from build123d import *

# Parameters (mm, degrees)
SKETCH_1_R          = 1.6
EXTRUDE_1_DEPTH     = 3
SKETCH_2_R          = 1.6
CUT_EXTRUDE_1_DEPTH = 4
SKETCH_3_R          = 1.6
CUT_EXTRUDE_2_DEPTH = 4
SKETCH_4_W          = 38
SKETCH_4_H          = 12.5
CUT_EXTRUDE_3_DEPTH = 4
FILLET_1_R          = 3


with BuildPart() as part:
    # 草图1 → 凸台-拉伸1 (new body)
    with BuildSketch(Plane.XY):
        Polygon((-40, 0), (-48, 25.855555556), (-48, 50), (5, 50), (5, 25.855555556), (0, 0), align=None)
        with Locations((-44, 46)):
            Circle(SKETCH_1_R, mode=Mode.SUBTRACT)
        with Locations((1, 46)):
            Circle(SKETCH_1_R, mode=Mode.SUBTRACT)
        with Locations((1, 27.5)):
            Circle(SKETCH_1_R, mode=Mode.SUBTRACT)
        with Locations((-44, 27.5)):
            Circle(SKETCH_1_R, mode=Mode.SUBTRACT)
    extrude(amount=EXTRUDE_1_DEPTH)

    # 草图2 → 切除-拉伸1 (cut, through all)
    with BuildSketch(Plane.XY.offset(3)):
        with Locations((-5, 3)):
            Circle(SKETCH_2_R)
        with Locations((-15, 3)):
            Circle(SKETCH_2_R)
        with Locations((-25, 3)):
            Circle(SKETCH_2_R)
        with Locations((-35, 3)):
            Circle(SKETCH_2_R)
    extrude(amount=-CUT_EXTRUDE_1_DEPTH, mode=Mode.SUBTRACT)

    # 草图3 → 切除-拉伸2 (cut, through all)
    with BuildSketch(Plane.XY.offset(3)):
        with Locations((-13.5, 10)):
            Circle(SKETCH_3_R)
        with Locations((-21.5, 10)):
            Circle(SKETCH_3_R)
        with Locations((-33.5, 10)):
            Circle(SKETCH_3_R)
        with Locations((-21.5, 34)):
            Circle(SKETCH_3_R)
    extrude(amount=-CUT_EXTRUDE_2_DEPTH, mode=Mode.SUBTRACT)

    # 草图4 → 切除-拉伸3 (cut, through all)
    with BuildSketch(Plane.XY.offset(3)):
        with Locations((-21.5, 36.75)):
            Rectangle(SKETCH_4_W, SKETCH_4_H)
    extrude(amount=-CUT_EXTRUDE_3_DEPTH, mode=Mode.SUBTRACT)

    # 圆角1
    fillet_1_edges = [part.edges().sort_by_distance(p)[0] for p in [
        (0, 0, 1.5),
        (-40, 0, 1.5),
        (-48, 25.855555556, 1.5),
        (-48, 50, 1.5),
        (5, 50, 1.5),
        (5, 25.855555556, 1.5),
        (-2.5, 43, 1.5),
        (-2.5, 30.5, 1.5),
        (-40.5, 30.5, 1.5),
        (-40.5, 43, 1.5),
    ]]
    fillet(fillet_1_edges, radius=FILLET_1_R)


solid = part.part
CAD build for the part. Positions are in the model's coordinates, mm. A direction names the side the tool comes from. Round coordinates to 2 decimals unless told otherwise and drop trailing zeros. Order: outer loops, then holes, each group sorted by start corner. A loop starts at its lowest first (then second) coordinate and runs counter-clockwise, first axis right, second up. Notation, with made-up numbers: (-22, 51) - (4, 51) arc R21 cw to (4, 64) - close; hole circle Ø1 at (-32.75, -7.75). An arc over 180 degrees is marked (long way). Return JSON: item names as keys, results as strings.
(1) Tool access for faces 4 (the face through (-0.589, 0.668, 1.521)), 5 (the face through (-39.6, 31.36, 1.48)): list every direction of +Z, -Z, +X, -X, +Y, -Y with a clear straight run to the whole face (end or side of a thin tool).
Answer key:
{"face 4": "+Z, -Z, +X, -Y", "face 5": "+Z, -Z"}
(2) Cut at B-B (z = 2.5). State how many separate pieces and enclosed holes the cut face has, then the cut area to 3 significant figures.
Answer key:
{"separate pieces": "1", "enclosed holes": "12", "area": "1,920 mm^2"}
(3) Cut at C-C (x = -44). Give the cut face in (y, z), then the cut area to 3 significant figures.
Answer key:
{"outline": "(12.93, 0) - (25.9, 0) - (25.9, 3) - (12.93, 3) - close; (29.1, 0) - (44.4, 0) - (44.4, 3) - (29.1, 3) - close; (47.6, 0) - (50, 0) - (50, 3) - (47.6, 3) - close", "area": "92.0 mm^2"}
(4) Cut at A-A (x = -21). Give the cut face in (y, z), then the cut area to 3 significant figures.
Answer key:
{"outline": "(0, 0) - (8.48, 0) - (8.48, 3) - (0, 3) - close; (11.52, 0) - (30.5, 0) - (30.5, 3) - (11.52, 3) - close; (43, 0) - (50, 0) - (50, 3) - (43, 3) - close", "area": "103 mm^2"}
(5) Pull direction Y, two halves, no side cores. Call faces 1 (the face through (-22, 50, 1)), 2 (the face through (-35.1, 10.07, 1.52)), 3 (the face through (-48, 37, 1)): +Y half, -Y half, draft (parallel to the pull), parting line (faces both ways), or undercut.
Answer key:
{"face 1": "+Y half", "face 2": "undercut", "face 3": "draft"}
(6) Wall check: probe 1 along Y at (x, z) = (-19.5, 0.8); probe 2 along Y at (x, z) = (-34, 1.2); probe 3 along X at (y, z) = (34, 1.1). Give the ranges that are in metal, low to high. Write a range as from..to.
Answer key:
{"probe 1": "y = 0..30.5, 43..50", "probe 2": "y = 0..1.75, 4.25..8.48, 11.52..30.5, 43..50", "probe 3": "x = -48..-40.5, -2.5..5"}
(7) Pin check, flat tips, straight feed: pin 1 Ø5 at (x, y) = (-29, 8.5) entering from -Z; pin 2 Ø2.5 at (x, y) = (-13.5, 10) entering from +Z. Stop position of each tip, or through.
Answer key:
{"pin 1": "stops at z = 0", "pin 2": "passes through"}
